from build123d import *

# Parameters (mm, degrees)
SKETCH1_R           = 2.55
SKETCH1_R_2         = 1.69
SKETCH1_R_3         = 1.5
SKETCH1_W           = 12
SKETCH1_H           = 12
BOSS_EXTRUDE1_DEPTH = 3


with BuildPart() as part:
    # Sketch1 → Boss-Extrude1 (new body)
    with BuildSketch(Plane.XY):
        with BuildLine():
            Line((580.140809409, 26.062600666), (351.140809409, 26.062600666))
            ThreePointArc((351.140809409, 26.062600666), (349.019489066, 25.18392101), (348.140809409, 23.062600666))
            Line((348.140809409, 23.062600666), (348.140809409, -82.937399334))
            ThreePointArc((348.140809409, -82.937399334), (349.019489066, -85.058719677), (351.140809409, -85.937399334))
            Line((351.140809409, -85.937399334), (580.140809409, -85.937399334))
            ThreePointArc((580.140809409, -85.937399334), (582.262129753, -85.058719677), (583.140809409, -82.937399334))
            Line((583.140809409, -82.937399334), (583.140809409, 23.062600666))
            ThreePointArc((583.140809409, 23.062600666), (582.262129753, 25.18392101), (580.140809409, 26.062600666))
        make_face()
        with Locations((465.640809409, 8.562600666)):
            Circle(SKETCH1_R, mode=Mode.SUBTRACT)
        with Locations((465.640809409, -68.437399334)):
            Circle(SKETCH1_R, mode=Mode.SUBTRACT)
        with Locations((388.410230248, -45.355631642)):
            Circle(SKETCH1_R_2, mode=Mode.SUBTRACT)
        with Locations((413.759430248, -45.355631642)):
            Circle(SKETCH1_R_2, mode=Mode.SUBTRACT)
        with Locations((518.453126584, -30.412177954)):
            Circle(SKETCH1_R_3, mode=Mode.SUBTRACT)
        with Locations((558.453126584, -30.412177954)):
            Circle(SKETCH1_R_3, mode=Mode.SUBTRACT)
        with Locations((573.140809409, -29.937399334)):
            Circle(SKETCH1_R, mode=Mode.SUBTRACT)
        with Locations((358.140809409, -29.937399334)):
            Circle(SKETCH1_R, mode=Mode.SUBTRACT)
        with BuildLine():
            Line((405.862321678, -19.639380196), (405.862321678, -13.235418472))
            ThreePointArc((405.862321678, -13.235418472), (400.788140112, -10.437399334), (395.713958547, -13.235418472))
            Line((395.713958547, -13.235418472), (395.713958547, -19.639380196))
            ThreePointArc((395.713958547, -19.639380196), (400.788140112, -22.437399334), (405.862321678, -19.639380196))
        make_face(mode=Mode.SUBTRACT)
        with BuildLine():
            Line((482.140809409, 3.562600666), (449.140809409, 3.562600666))
            ThreePointArc((449.140809409, 3.562600666), (447.019489066, 2.68392101), (446.140809409, 0.562600666))
            Line((446.140809409, 0.562600666), (446.140809409, -60.437399334))
            ThreePointArc((446.140809409, -60.437399334), (447.019489066, -62.558719677), (449.140809409, -63.437399334))
            Line((449.140809409, -63.437399334), (482.140809409, -63.437399334))
            ThreePointArc((482.140809409, -63.437399334), (484.262129753, -62.558719677), (485.140809409, -60.437399334))
            Line((485.140809409, -60.437399334), (485.140809409, 0.562600666))
            ThreePointArc((485.140809409, 0.562600666), (484.262129753, 2.68392101), (482.140809409, 3.562600666))
        make_face(mode=Mode.SUBTRACT)
        with Locations((401.084830248, -45.355631642)):
            Rectangle(SKETCH1_W, SKETCH1_H, mode=Mode.SUBTRACT)
        with BuildLine():
            Line((551.953126584, 1.587822046), (524.953126584, 1.587822046))
            ThreePointArc((524.953126584, 1.587822046), (524.246019803, 1.294928827), (523.953126584, 0.587822046))
            Line((523.953126584, 0.587822046), (523.953126584, -61.412177954))
            ThreePointArc((523.953126584, -61.412177954), (524.246019803, -62.119284735), (524.953126584, -62.412177954))
            Line((524.953126584, -62.412177954), (551.953126584, -62.412177954))
            ThreePointArc((551.953126584, -62.412177954), (552.660233365, -62.119284735), (552.953126584, -61.412177954))
            Line((552.953126584, -61.412177954), (552.953126584, 0.587822046))
            ThreePointArc((552.953126584, 0.587822046), (552.660233365, 1.294928827), (551.953126584, 1.587822046))
        make_face(mode=Mode.SUBTRACT)
    extrude(amount=BOSS_EXTRUDE1_DEPTH)


solid = part.part
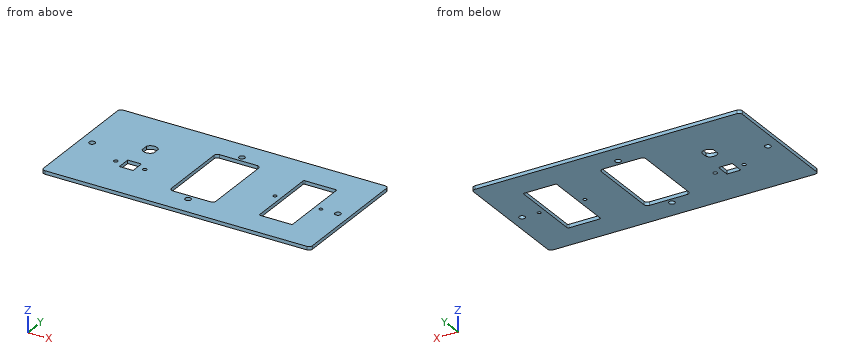
Design review of the part built by this model. Coordinates are the model's own, in mm. Coordinates: 2 decimals unless noted, no trailing zeros. Loops run counter-clockwise (first coordinate to the right, second up) from the corner with the lowest first, then second, coordinate; pieces in that order, holes last.
Item 1: Add section D-D (z = 1.8). Give the number of separate pieces and of enclosed holes in the cut face, and give its area (3 significant figures).
Completed:
separate pieces: 1
enclosed holes: 12
area: 21,500 mm2
Item 2: Wall thickness on L1, parallel to X at y = -16, z = 2.65; L2, parallel to X at y = 0, z = 1.3; L3, parallel to Y at x = 456, z = 2.35: over which ranges is each line inside the solid? List them lowest first.
Completed:
L1: x = 348.14 to 395.71, 405.86 to 446.14, 485.14 to 523.95, 552.95 to 583.14
L2: x = 348.14 to 446.14, 485.14 to 523.95, 552.95 to 583.14
L3: y = -85.94 to -63.44, 3.56 to 26.06
Item 3: Add section A-A (y = -55). Write out the cut boundary in (x, z).
Completed:
outline: (348.14, 0) - (446.14, 0) - (446.14, 3) - (348.14, 3) - close; (485.14, 0) - (523.95, 0) - (523.95, 3) - (485.14, 3) - close; (552.95, 0) - (583.14, 0) - (583.14, 3) - (552.95, 3) - close
Item 4: Add section C-C (x = 454). Write out the cut boundary in (y, z), and give its area (3 significant figures).
Completed:
outline: (-85.94, 0) - (-63.44, 0) - (-63.44, 3) - (-85.94, 3) - close; (3.56, 0) - (26.06, 0) - (26.06, 3) - (3.56, 3) - close
area: 135 mm2
Item 5: Add section B-B (x = 543.5). Write out the cut boundary in (y, z), and give its area (3 significant figures).
Completed:
outline: (-85.94, 0) - (-62.41, 0) - (-62.41, 3) - (-85.94, 3) - close; (1.59, 0) - (26.06, 0) - (26.06, 3) - (1.59, 3) - close
area: 144 mm2
